Job drawing, mm, ordinate dimensions from the low corner. One solid piece. A direction names the side the tool comes from. Round coordinates to 2 decimals unless told otherwise and drop trailing zeros. Loops run counter-clockwise (first coordinate to the right, second up) from the corner with the lowest first, then second, coordinate; pieces in that order, holes last.
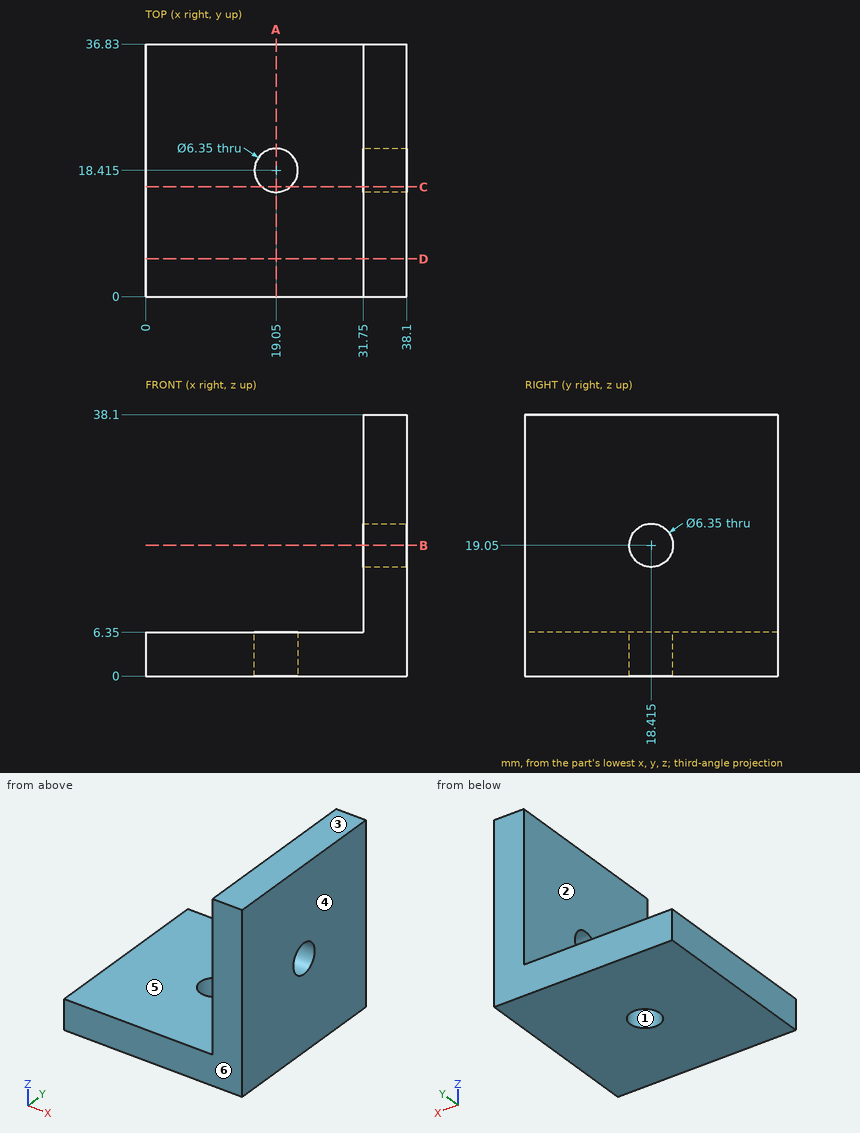
1) Slice it at D-D, the plane y = 5.5. Give the cut face in (x, z).
Values:
outline: (0, 0) - (38.1, 0) - (38.1, 38.1) - (31.75, 38.1) - (31.75, 6.35) - (0, 6.35) - close
2) Slice it at B-B, the plane z = 19.05. Give the cut face in (x, y), then the cut area to 3 significant figures.
Values:
outline: (31.75, 0) - (38.1, 0) - (38.1, 15.24) - (31.75, 15.24) - close; (31.75, 21.59) - (38.1, 21.59) - (38.1, 36.83) - (31.75, 36.83) - close
area: 194 mm2
3) Tool access for the marked faces 5 and 6: list every direction of +Z, -Z, +X, -X, +Y, -Y with a clear straight run to the whole face (end or side of a thin tool).
Values:
face 5: +Z, -X, +Y, -Y
face 6: +Z, -Z, +X, -X, -Y
4) Slice it at A-A, the plane x = 19.05. Give the cut face in (y, z), then the cut area to 3 significant figures.
Values:
outline: (0, 0) - (15.24, 0) - (15.24, 6.35) - (0, 6.35) - close; (21.59, 0) - (36.83, 0) - (36.83, 6.35) - (21.59, 6.35) - close
area: 194 mm2
5) Drop flat-ended pins along their axis: pin 1 Ø12 at (y, z) = (17, 25) entering from -X; pin 2 Ø1.5 at (x, y) = (20.5, 22.5) entering from +Z; pin 3 Ø8 at (x, y) = (25.5, 20.5) entering from +Z. Give the stop position or say it passes through.
Values:
pin 1: stops at x = 31.75
pin 2: stops at z = 6.35
pin 3: stops at z = 6.35
6) Wall check: line 1 along Y through (x, z) = (36, 19); line 2 along X through (y, z) = (8.5, 19.5); line 3 along Z through (x, y) = (7.5, 5). Give the ranges that are in metal, low to high.
Values:
line 1: y = 0 to 15.24, 21.59 to 36.83
line 2: x = 31.75 to 38.1
line 3: z = 0 to 6.35
7) Mould opens along X. For the marked faces 1, 2, 3 and 4 say: released by +X, released by -X, zero draft, split by the parting line, or undercut.
Values:
face 1: undercut
face 2: released by -X
face 3: zero draft
face 4: released by +X
8) Slice it at C-C, the plane y = 16. Give the cut face in (x, z), then the cut area to 3 significant figures.
Values:
outline: (0, 0) - (16.99, 0) - (16.99, 6.35) - (0, 6.35) - close; (21.11, 0) - (38.1, 0) - (38.1, 16.99) - (31.75, 16.99) - (31.75, 6.35) - (21.11, 6.35) - close; (31.75, 21.11) - (38.1, 21.11) - (38.1, 38.1) - (31.75, 38.1) - close
area: 391 mm2
